Source: CAD feature listing. Evaluate the final solid. Frame: model axes, mm. A direction names the side the tool comes from. Round coordinates to 2 decimals unless told otherwise and drop trailing zeros. Order: outer loops, then holes, each group sorted by start corner. A loop starts at its lowest first (then second) coordinate and runs counter-clockwise, first axis right, second up. Notation, with made-up numbers: M 64.25,19.25 L 72.25,19.25 A27 ccw 72.25,36.25 Z; hole C 55,63.5 d11. An arc over 180 degrees is marked long. Answer as CSV lines item,"result". Start each with the question number.
Item 1: Section query A-A on x = 39.5. Return the cut outline in (y, z).
Item 2: Pull-direction query (Z, two-part tool) for faces 4 (the face through (27.85, -9, 3)), 5 (the face through (-1, 0, 0)), 6 (the face through (31.4, -9, 5)); classes: +Z half, -Z half, draft (parallel to the pull), parting line (faces both ways), or undercut.
Item 3: Line query: line 1 (X direction, y = -12, z = 5.5); line 2 (X direction, y = -13, z = 4.75); line 3 (Z direction, x = 14, y = 1.5). Output: solid intervals per line, ascending. Write a range as [from, to].
Item 4: First-contact query: P1, Ø1.1, axis at x = -31, z = 5, coming from the -Y side; P2, Ø1, axis at y = -17.5, z = 3.5, coming from the +X side; P3, Ø10, axis at x = 2.5, y = 12, coming from the +Z side; P4, Ø0.6, axis at y = -8, z = 3.5, coming from the -X side. Flat tips, straight axial feed; report the tip coordinate or a pass-through.
Item 5: Section query B-B on y = 1. Return the cut outline in (x, z).
Item 6: Set-up query: faces 1 (the face through (-30, -11.05, 3)), 2 (the face through (32.18, -5.42, 3.49)), 3 (the face through (-30, -6.45, 3)). Return all of +Z, -Z, +X, -X, +Y, -Y with unobstructed straight access to the full face (end or side cutting, diameter ignored); none if empty.
from build123d import *

# Parameters (mm, degrees)
SKETCH_W      = 102
SKETCH_H      = 48
PAD_DEPTH     = 2.5
PAD001_DEPTH  = 2
PAD002_DEPTH  = 2
SKETCH004_W   = 10
SKETCH004_H   = 2.5
SKETCH004_W_2 = 2.5
SKETCH004_H_2 = 10
POCKET_DEPTH  = 4
CHAMFER_SIZE  = 1


with BuildPart() as part:
    # Sketch → Pad (new body)
    with BuildSketch(Plane.XY):
        Rectangle(SKETCH_W, SKETCH_H)
    extrude(amount=PAD_DEPTH)

    # Sketch001 (on Face6 of Pad) → Pad001 (join)
    with BuildSketch(Plane.XY.offset(2.5)):
        with BuildLine():
            ThreePointArc((-32.395, -6.45), (-34.695, -8.75), (-32.395, -11.05))
            Line((-32.395, -11.05), (-27.905, -11.05))
            ThreePointArc((-27.905, -11.05), (-25.605, -8.75), (-27.905, -6.45))
            Line((-32.395, -6.45), (-27.905, -6.45))
        make_face()
        with BuildLine():
            ThreePointArc((32.45, -6.505), (30.15, -4.205), (27.85, -6.505))
            Line((27.85, -6.505), (27.85, -10.995))
            ThreePointArc((27.85, -10.995), (30.15, -13.295), (32.45, -10.995))
            Line((32.45, -6.505), (32.45, -10.995))
        make_face()
    extrude(amount=PAD001_DEPTH)

    # Sketch002 (on Face15 of Pad001) → Pad002 (join)
    with BuildSketch(Plane.XY.offset(4.5)):
        with BuildLine():
            ThreePointArc((-32.395, -6.048796), (-35.096204, -8.75), (-32.395, -11.451204))
            Line((-32.395, -11.451204), (-27.905, -11.451204))
            ThreePointArc((-27.905, -11.451204), (-25.203796, -8.75), (-27.905, -6.048796))
            Line((-32.395, -6.048796), (-27.905, -6.048796))
        make_face()
        with BuildLine():
            ThreePointArc((32.65, -6.505), (30.15, -4.005), (27.65, -6.505))
            Line((27.65, -6.505), (27.65, -10.995))
            ThreePointArc((27.65, -10.995), (30.15, -13.495), (32.65, -10.995))
            Line((32.65, -6.505), (32.65, -10.995))
        make_face()
    extrude(amount=PAD002_DEPTH)

    # Sketch004 (on Face25 of Pad002) → Pocket (cut)
    with BuildSketch(Plane.XY.offset(6.5)):
        with Locations((-30.15, -8.75)):
            Rectangle(SKETCH004_W, SKETCH004_H)
        with Locations((30.15, -8.75)):
            Rectangle(SKETCH004_W_2, SKETCH004_H_2)
    extrude(amount=-POCKET_DEPTH, mode=Mode.SUBTRACT)

    # Chamfer
    chamfer_edges = [part.edges().sort_by_distance(p)[0] for p in [
        (-33.795, -6.439912, 6.5),
        (-30.15, -6.048796, 6.5),
        (-26.505, -6.439912, 6.5),
        (-26.505, -11.060088, 6.5),
        (-30.15, -11.451204, 6.5),
        (-33.795, -11.060088, 6.5),
        (27.984936, -5.255, 6.5),
        (27.65, -8.75, 6.5),
        (27.984936, -12.245, 6.5),
        (32.315064, -12.245, 6.5),
        (32.65, -8.75, 6.5),
        (32.315064, -5.255, 6.5),
    ]]
    chamfer(chamfer_edges, length=CHAMFER_SIZE)


solid = part.part
Results:
1,outline,"M -24,0 L 24,0 L 24,2.5 L -24,2.5 Z"
2,face 4,"undercut"
2,face 5,"-Z half"
2,face 6,"draft"
3,line 1,"[27.86, 28.9], [31.4, 32.44]"
3,line 2,"[28.66, 28.9], [31.4, 31.64]"
3,line 3,"[0, 2.5]"
4,P1,"y = -11.45"
4,P2,"through"
4,P3,"z = 2.5"
4,P4,"x = 27.85"
5,outline,"M -51,0 L 51,0 L 51,2.5 L -51,2.5 Z"
6,face 1,"-X, -Y"
6,face 2,"+X, +Y"
6,face 3,"-X, +Y"
